For this review, take the finished solid that the model builds, in its own axes (mm). Face numbers are marked on the shaded views. A direction names the side the tool comes from. Give positions to 0.01 mm unless a question says otherwise; leave off trailing zeros. Loops run counter-clockwise (first coordinate to the right, second up) from the corner with the lowest first, then second, coordinate; pieces in that order, holes last. Notation, with made-up numbers: (67, 4) - (96, 4) arc R23 cw to (96, 36) - close; hole circle Ø3 at (8, 54). An arc over 180 degrees is marked (long way). Put each result on its own line as item: value. Start each with the question number.
from build123d import *

# Parameters (mm, degrees)
CUT_EXTRUDE1_DEPTH       = 8
CIRPATTERN1_COUNT        = 3
CUT_EXTRUDE2_DEPTH       = 13
FILLET1_R                = 2
CUT_EXTRUDE3_REACH       = 125.655
SKETCH6_R                = 3
CIRPATTERN2_COUNT        = 3
FILLET1_OF_CIRPATTERN2_R = 2
CUT_EXTRUDE4_DEPTH       = 30
FILLET2_R                = 1
CIRPATTERN3_COUNT        = 3
FILLET2_OF_CIRPATTERN3_R = 1
CUT_EXTRUDE5_REACH       = 130.22
SKETCH9_W                = 102
SKETCH9_H                = 12
CHAMFER2_SIZE            = 2


with BuildPart() as part:
    # Sketch1 → Revolve1 (revolve)
    with BuildSketch(Plane.XY, mode=Mode.PRIVATE) as revolve1_sk:
        Polygon((0, 20), (0, 42.5), (-55, 42.5), (-55, 40.5), (-57, 40.5), (-57, 42.5), (-72, 42.5), (-72, 37.6), (-102, 37.6), (-102, 20), align=None)
    revolve(revolve1_sk.sketch.rotate(Axis((-534.701035213, 0, 0), (1, 0, 0)), 90), axis=Axis((-534.701035213, 0, 0), (1, 0, 0)))

    # Sketch3 → Cut-Extrude1 (cut, symmetric)
    with BuildSketch(Plane.XY):
        with BuildLine():
            Line((-102, 24.5), (-42, 24.5))
            ThreePointArc((-42, 24.5), (-24.11145618, 28.72291236), (-10, 40.5))
            Line((-10, 40.5), (0, 40.5))
            Line((0, 40.5), (0, 42.5))
            Line((0, 42.5), (-55, 42.5))
            Line((-55, 42.5), (-55, 40.5))
            Line((-55, 40.5), (-57, 40.5))
            Line((-57, 40.5), (-57, 42.5))
            Line((-57, 42.5), (-72, 42.5))
            Line((-72, 42.5), (-72, 37.6))
            Line((-72, 37.6), (-102, 37.6))
            Line((-102, 37.6), (-102, 24.5))
        make_face()
    cut_extrude1 = extrude(amount=CUT_EXTRUDE1_DEPTH, both=True, mode=Mode.SUBTRACT)

    # CirPattern1: Cut-Extrude1 ×3 about axis
    cirpattern1_axis = Axis((0, 0, 0), (1, 0, 0))
    for i in range(1, CIRPATTERN1_COUNT):
        add(cut_extrude1.rotate(cirpattern1_axis, i * 360 / CIRPATTERN1_COUNT), mode=Mode.SUBTRACT)

    # Sketch4 → Cut-Extrude2 (cut)
    with BuildSketch(Plane.ZY.offset(102)):
        with BuildLine():
            Line((-13, 35.281156444), (-13, 24.5))
            Line((-13, 24.5), (-28.522096697, 24.5))
            ThreePointArc((-28.522096697, 24.5), (-21.449462979, 30.881718506), (-13, 35.281156444))
        make_face()
        with BuildLine():
            Line((13, 35.281156444), (13, 24.5))
            Line((13, 24.5), (28.522096697, 24.5))
            ThreePointArc((28.522096697, 24.5), (21.449462979, 30.881718506), (13, 35.281156444))
        make_face()
    cut_extrude2 = extrude(amount=-CUT_EXTRUDE2_DEPTH, mode=Mode.SUBTRACT)

    # Fillet1
    fillet1_edges = [part.edges().sort_by_distance(p)[0] for p in [
        (-89, 29.890578222, -13),
        (-89, 29.890578222, 13),
    ]]
    fillet(fillet1_edges, radius=FILLET1_R)

    # Cut-Extrude3: up to this face of the body (flat: up to its plane)
    cut_extrude3_end = Plane(part.part.faces().sort_by_distance((-96.5, 29.890578222, -13))[0])
    # Sketch6 → Cut-Extrude3 (cut, up to the picked face)
    with BuildSketch(Plane.XY.offset(13), mode=Mode.PRIVATE) as cut_extrude3_sk1:
        with Locations((-96.5, 30.5)):
            Circle(SKETCH6_R)
    cut_extrude3_tool1 = split(extrude(cut_extrude3_sk1.sketch, amount=-CUT_EXTRUDE3_REACH, mode=Mode.PRIVATE), bisect_by=cut_extrude3_end, keep=Keep.BOTH, mode=Mode.PRIVATE)
    cut_extrude3 = cut_extrude3_tool1.solids().sort_by(Axis((-96.5, 30.5, 13), (0, 0, -1)))[0]
    add(cut_extrude3, mode=Mode.SUBTRACT)

    # CirPattern2: Cut-Extrude2, Cut-Extrude3 ×3 about axis
    cirpattern2_axis = Axis((0, 0, 0), (1, 0, 0))
    add([cut_extrude2.rotate(cirpattern2_axis, i * 360 / CIRPATTERN2_COUNT) for i in range(1, CIRPATTERN2_COUNT)], mode=Mode.SUBTRACT)
    add([cut_extrude3.rotate(cirpattern2_axis, i * 360 / CIRPATTERN2_COUNT) for i in range(1, CIRPATTERN2_COUNT)], mode=Mode.SUBTRACT)

    # Fillet1 of CirPattern2
    fillet1_of_cirpattern2_edges = [part.edges().sort_by_distance(p)[0] for p in [
        (-89, -3.686958862, 32.386000074),
        (-89, -26.20361936, 19.386000074),
        (-89, -26.20361936, -19.386000074),
        (-89, -3.686958862, -32.386000074),
    ]]
    fillet(fillet1_of_cirpattern2_edges, radius=FILLET1_OF_CIRPATTERN2_R)

    # Sketch7 → Cut-Extrude4 (cut)
    with BuildSketch(Plane.ZY.offset(102)):
        with BuildLine():
            Line((-6, -37.118189611), (-6, -32.3))
            Line((-6, -32.3), (6, -32.3))
            Line((6, -32.3), (6, -37.118189611))
            ThreePointArc((6, -37.118189611), (0, -37.6), (-6, -37.118189611))
        make_face()
    cut_extrude4 = extrude(amount=-CUT_EXTRUDE4_DEPTH, mode=Mode.SUBTRACT)

    # Fillet2
    fillet2_edges = [part.edges().sort_by_distance(p)[0] for p in [
        (-87, -37.118189611, 6),
        (-87, -37.118189611, -6),
    ]]
    fillet(fillet2_edges, radius=FILLET2_R)

    # CirPattern3: Cut-Extrude4 ×3 about axis
    cirpattern3_axis = Axis((0, 0, 0), (1, 0, 0))
    for i in range(1, CIRPATTERN3_COUNT):
        add(cut_extrude4.rotate(cirpattern3_axis, i * 360 / CIRPATTERN3_COUNT), mode=Mode.SUBTRACT)

    # Fillet2 of CirPattern3
    fillet2_of_cirpattern3_edges = [part.edges().sort_by_distance(p)[0] for p in [
        (-87, 13.362942383, -35.145295146),
        (-87, 23.755247228, -29.145295146),
        (-87, 23.755247228, 29.145295146),
        (-87, 13.362942383, 35.145295146),
    ]]
    fillet(fillet2_of_cirpattern3_edges, radius=FILLET2_OF_CIRPATTERN3_R)

    # Sketch9 → Cut-Extrude5 (cut, up to next)
    with BuildSketch(Plane(origin=(0, -23.3, 0), x_dir=(1, 0, 0), z_dir=(0, 1, 0)), mode=Mode.PRIVATE) as cut_extrude5_sk1:
        with Locations((-51, 0)):
            Rectangle(SKETCH9_W, SKETCH9_H)
    cut_extrude5_tool1 = extrude(cut_extrude5_sk1.sketch, amount=CUT_EXTRUDE5_REACH, mode=Mode.PRIVATE) & part.part
    add(cut_extrude5_tool1.solids().sort_by_distance((-51, -23.3, 0))[0], mode=Mode.SUBTRACT)

    # Chamfer2
    chamfer2_edges = [part.edges().sort_by_distance(p)[0] for p in [
        (0, 20, 0),
        (-102, 20, 0),
    ]]
    chamfer(chamfer2_edges, length=CHAMFER2_SIZE)


solid = part.part
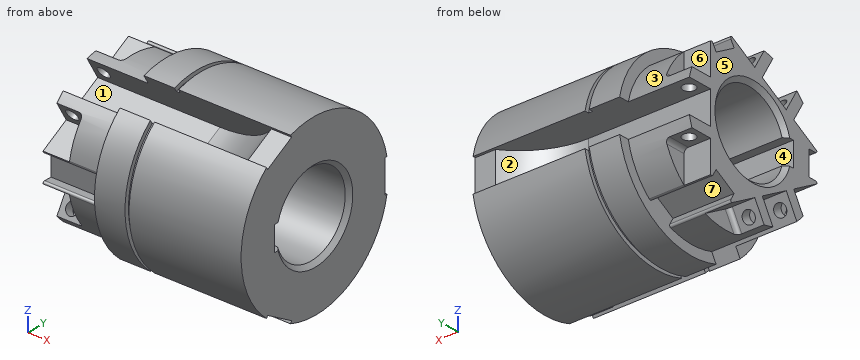
1) Take a section at A-A on z = 0. State the section outline as (x, y) points, and give its area (3 significant figures).
2) Machinability: for the marked faces 1, 2 and 3, which of the approach directions +Z, -Z, +X, -X, +Y, -Y give a long, thin tool a straight path to every point of the face, cutting with its end or side? Answer none if there is none.
3) Take a section at C-C on y = 30.5. State how many separate pieces and enclosed holes the cut face has, and give its area (3 significant figures).
4) Insertion check: P1, Ø6, axis at x = -88, z = -1.5, coming from the -Y side; P2, Ø2, axis at x = -41, y = -21, coming from the +Z side; P3, Ø6, axis at x = -31, y = -13, coming from the -Z side. Each pin has a flat end and moves straight along its axis. Give the tip position at first contact, or say it passes through.
5) Wall thickness on probe 1 along Y at (x, z) = (-96.5, -10.5); probe 2 along Y at (x, z) = (-42, 0); probe 3 along Y at (x, z) = (-96, -11): over which ranges is each line inside the solid? List them lowest first.
6) Take a section at B-B on x = -62. State the section outline as (y, z) points, and give its area (3 significant figures).
7) Mouldability with a two-part tool opening along Y and no side actions: class the marked faces 4, 5, 6 and 7 as released by +Y, released by -Y, zero draft, split by the parting line, or undercut.
Answers follow:
1. outline: (-102, -32.3) - (-72, -32.3) - (-72, -42.5) - (-57, -42.5) - (-57, -40.5) - (-55, -40.5) - (-55, -42.5) - (0, -42.5) - (0, -23.3) - (-102, -23.3) - close; (-102, 22) - (-100, 20) - (-2, 20) - (0, 22) - (0, 40.5) - (-10, 40.5) arc R40 cw to (-42, 24.5) - (-102, 24.5) - close
1. area: 2,420 mm2
2. face 1: -X
2. face 2: -X, +Y
2. face 3: +Z, -X, +Y
3. separate pieces: 3
3. enclosed holes: 0
3. area: 3,980 mm2
4. P1: y = -32.3
4. P2: z = 22.11
4. P3: z = -41.31
5. probe 1: -30.81 to -17.02, 17.02 to 27.5, 33.5 to 36.1
5. probe 2: -42.5 to -23.3, 20 to 24.5
5. probe 3: -29.95 to -16.7, 16.7 to 27.54, 33.46 to 35.95
6. outline: (-27.8, -32.15) - (-19.18, -17.22) - (-5.32, -25.22) - (-13.94, -40.15) arc R42.5 ccw to (41.74, -8) - (24.5, -8) - (24.5, 8) - (41.74, 8) arc R42.5 ccw to (-13.94, 40.15) - (-5.32, 25.22) - (-19.18, 17.22) - (-27.8, 32.15) arc R42.5 ccw to start; hole (-23.3, -6) - (-19.08, -6) arc R20 ccw (long way) to (-19.08, 6) - (-23.3, 6) - close
6. area: 3,520 mm2
7. face 4: undercut
7. face 5: zero draft
7. face 6: released by +Y
7. face 7: undercut
